The model under review builds one solid part; all positions refer to its coordinate system, in mm. A direction names the side the tool comes from. Give positions to 0.01 mm unless a question says otherwise; leave off trailing zeros. Order: outer loops, then holes, each group sorted by start corner. A loop starts at its lowest first (then second) coordinate and runs counter-clockwise, first axis right, second up. Notation, with made-up numbers: (40, 33.25) - (49, 33.25) arc R30 ccw to (49, 60.25) - close; hole circle Ø5 at (31.5, 6.25). An arc over 180 degrees is marked (long way). Put each result on its own line as item: value.
```python
from build123d import *

# Parameters (mm, degrees)
F1_DEPTH = 50
F2_T     = 3
F4_DEPTH = 50


# Not quite as in the source:
# - a shell that OpenCascade refuses in one call is made with other operations: the cavity is built on its own and cut out


with BuildPart() as f1:
    # F0 (on Right) → F1 (new body)
    with BuildSketch(Plane.YZ):
        with BuildLine():
            Line((-2.5980762114, 57.9554029985), (-54.0879656003, -31.2277014993))
            Line((-54.0879656003, -31.2277014993), (48.8918131776, -31.2277014993))
            ThreePointArc((48.8918131776, -31.2277014993), (51.4898893889, -29.7277014993), (51.4898893889, -26.7277014993))
            Line((51.4898893889, -26.7277014993), (2.5980762114, 57.9554029985))
            ThreePointArc((2.5980762114, 57.9554029985), (0, 59.4554029985), (-2.5980762114, 57.9554029985))
        make_face()
    extrude(amount=F1_DEPTH)

    # F2: shell of thickness 3, made by hand


with BuildPart() as f2_core1:
    # F2_t2: copy of F1
    add(f1.part)

    # the walls: a layer under each face that stays
    f2_faces = [f2_core1.faces().sort_by_distance(p)[0] for p in [
        (25, -28.3430209058, 13.3638507496),
        (25, -2.5980762114, -31.2277014993),
        (25, 27.0439828001, 15.6138507496),
    ]]
    thicken(f2_faces, amount=-F2_T, mode=Mode.SUBTRACT)


with BuildPart() as f1_1:
    add(f1.part)

    # what is left inside the walls is the cavity
    f2_cavity = [f2_core1.part.solids().sort_by_distance(p)[0] for p in [
        (33.333333, -24.419926, 14.098851),
    ]]
    add(f2_cavity, mode=Mode.SUBTRACT)

    # F3 (on Right) → F4 (join)
    with BuildSketch(Plane.YZ):
        with BuildLine():
            Line((-54.0879656003, -31.2277014993), (-52.5466056017, -28.5579876689))
            Line((-52.5466056017, -28.5579876689), (-62.9389104471, -22.5579876689))
            Line((-62.9389104471, -22.5579876689), (-60.3408342357, -18.0579876689))
            Line((-60.3408342357, -18.0579876689), (-62.0728850433, -17.0579876689))
            ThreePointArc((-62.0728850433, -17.0579876689), (-62.8317040884, -16.9580872464), (-63.4389104471, -17.4240130727))
            Line((-63.4389104471, -17.4240130727), (-68.8103974646, -26.7277014993))
            ThreePointArc((-68.8103974646, -26.7277014993), (-68.8103974646, -29.7277014993), (-66.2123212533, -31.2277014993))
            Line((-66.2123212533, -31.2277014993), (-54.0879656003, -31.2277014993))
        make_face()
    extrude(amount=F4_DEPTH)


solid = f1_1.part
```
(1) Take a section at B-B, the plane z = 0. Write out the cut boundary in (x, y), then the cut area to 3 significant figures.
The answers:
outline: (0, -36.06) - (50, -36.06) - (50, -32.59) - (0, -32.59) - close; (0, 32.59) - (50, 32.59) - (50, 36.06) - (0, 36.06) - close
area: 346 mm^2
(2) Wall thickness on L1, parallel to Y at x = 36.5, z = -20.5; L2, parallel to Y at x = 40, z = -3; L3, parallel to Y at x = 3, z = 39: over which ranges is each line inside the solid? List them lowest first.
The answers:
L1: -65.21 to -61.75, -47.89 to -44.43, 44.43 to 47.89
L2: -37.79 to -34.33, 34.33 to 37.79
L3: -13.54 to -10.08, 10.08 to 13.54
(3) Clearance check with flat-ended pins moving along their axes: pin 1 Ø1.5 at (x, y) = (16, -53) entering from +Z; pin 2 Ø8 at (x, y) = (34, -15.5) entering from +Z; pin 3 Ø1.5 at (x, z) = (17.5, 48) entering from +Y. State where each tip first meets the part, or that it passes through.
The answers:
pin 1: z = -27.86
pin 2: z = 42.54
pin 3: y = 8.78
(4) The part is to be moulded in two halves that separate along Y. For faces 1 (the flat face through (24.6, 27.4, 15)), 2 (the cylindrical face through (24.65, 0.044, 59.455)), 3 (the flat face through (24.65, -24.1, 14.71)), say which applies: pulls with the +Y half, pulls with the -Y half, needs draft (parallel to the pull), parting line crosses it, or undercut.
The answers:
face 1: pulls with the +Y half
face 2: parting line crosses it
face 3: undercut
(5) Take a section at A-A, the plane x = 23. Write out the cut boundary in (y, z), then the cut area to 3 significant figures.
The answers:
outline: (-68.81, -26.73) arc R3 ccw to (-66.21, -31.23) - (48.89, -31.23) arc R3 ccw to (51.49, -26.73) - (2.6, 57.96) arc R3 ccw to (-2.6, 57.96) - (-52.55, -28.56) - (-62.94, -22.56) - (-60.34, -18.06) - (-62.07, -17.06) arc R1 ccw to (-63.44, -17.42) - close; hole (-48.89, -28.23) - (48.89, -28.23) - (0, 56.46) - close
area: 1,030 mm^2
(6) For faces 4 (the flat face through (24.6, 24.8, 13.5)), 5 (the flat face through (50, -27, 11)), list the 3-axis set-ups (+Z, -Z, +X, -X, +Y, -Y) from which the entire face can be reached by the end or side of a thin tool; tool diameter is ignored.
The answers:
face 4: +X, -X
face 5: +Z, -Z, +X, +Y, -Y
(7) Take a section at C-C, the plane y = -6. Write out the cut boundary in (x, z), then the cut area to 3 significant figures.
The answers:
outline: (0, -31.23) - (50, -31.23) - (50, -28.23) - (0, -28.23) - close; (0, 46.06) - (50, 46.06) - (50, 52.06) - (0, 52.06) - close
area: 450 mm^2
